Read the model definition and answer for the solid it produces. Units are mm, in the model's axes. Face numbers are marked on the shaded views. A direction names the side the tool comes from. Coordinates: 2 decimals unless noted, no trailing zeros. Write each loop counter-clockwise with the first axis right and the second up, starting at its lowest first coordinate (ties: lowest second). Pieces come first, ordered by that corner, then holes. Notation, with made-up numbers: M 41,-21 L 82,-21 A22 cw 82,9 Z; hole C -19,-14 d5. An arc over 180 degrees is marked long. Use a Markdown table: item, result. Add a question column.
from build123d import *

# Parameters (mm, degrees)
SKETCH1_W                 = 71
SKETCH1_H                 = 250
BOSS_EXTRUDE1_DEPTH       = 5
SKETCH2_W                 = 65
SKETCH2_H                 = 45
BOSS_EXTRUDE3_DEPTH       = 2
LPATTERN1_COUNT           = 3
LPATTERN1_PITCH           = 50
SKETCH3_W                 = 69
SKETCH3_H                 = 48.754858224
BOSS_EXTRUDE8_DEPTH       = 25
LPATTERN5_COUNT           = 3
LPATTERN5_PITCH           = 50
LPATTERN6_COUNT           = 3
LPATTERN6_PITCH           = 70
LPATTERN6_COPY_1_SKETCH_W = 65
LPATTERN6_COPY_1_SKETCH_H = 45
LPATTERN6_COPY_1_DEPTH    = 2
LPATTERN6_COPY_2_SKETCH_W = 65
LPATTERN6_COPY_2_SKETCH_H = 45
LPATTERN6_COPY_2_DEPTH    = 2
LPATTERN6_COPY_3_SKETCH_W = 65
LPATTERN6_COPY_3_SKETCH_H = 45
LPATTERN6_COPY_3_DEPTH    = 2
LPATTERN6_COPY_4_SKETCH_W = 65
LPATTERN6_COPY_4_SKETCH_H = 45
LPATTERN6_COPY_4_DEPTH    = 2
LPATTERN6_COPY_5_SKETCH_W = 69
LPATTERN6_COPY_5_SKETCH_H = 48.754858224
LPATTERN6_COPY_5_DEPTH    = 25
LPATTERN6_COPY_6_SKETCH_W = 69
LPATTERN6_COPY_6_SKETCH_H = 48.754858224
LPATTERN6_COPY_6_DEPTH    = 25
LPATTERN6_COPY_7_SKETCH_W = 69
LPATTERN6_COPY_7_SKETCH_H = 48.754858224
LPATTERN6_COPY_7_DEPTH    = 25
LPATTERN6_COPY_8_SKETCH_W = 69
LPATTERN6_COPY_8_SKETCH_H = 48.754858224
LPATTERN6_COPY_8_DEPTH    = 25
SKETCH6_W                 = 211
SKETCH6_H                 = 98.778316014
CUT_EXTRUDE1_DEPTH        = 10


with BuildPart() as part:
    # Sketch1 → Boss-Extrude1 (new body)
    with BuildSketch(Plane(origin=(0, 0, 0), x_dir=(1, 0, 0), z_dir=(0, 1, 0))):
        Rectangle(SKETCH1_W, SKETCH1_H)
    boss_extrude1 = extrude(amount=BOSS_EXTRUDE1_DEPTH)

    # Sketch2 → Boss-Extrude3 (add)
    with BuildSketch(Plane(origin=(0, 5, 0), x_dir=(1, 0, 0), z_dir=(0, 1, 0))):
        with Locations((0, -100)):
            Rectangle(SKETCH2_W, SKETCH2_H)
    boss_extrude3 = extrude(amount=BOSS_EXTRUDE3_DEPTH)

    # LPattern1: Boss-Extrude3 ×3
    with Locations(*[(0, 0, -i * LPATTERN1_PITCH) for i in range(1, LPATTERN1_COUNT)]):
        add(boss_extrude3)

    # Sketch3 → Boss-Extrude8 (add)
    with BuildSketch(Plane(origin=(0, 7, 0), x_dir=(1, 0, 0), z_dir=(0, 1, 0))):
        with Locations((0, -99.635002086)):
            Rectangle(SKETCH3_W, SKETCH3_H)
    boss_extrude8 = extrude(amount=BOSS_EXTRUDE8_DEPTH)

    # LPattern5: Boss-Extrude8 ×3
    with Locations(*[(0, 0, -i * LPATTERN5_PITCH) for i in range(1, LPATTERN5_COUNT)]):
        add(boss_extrude8)

    # LPattern6: Boss-Extrude1, Boss-Extrude3, Boss-Extrude8 ×3
    with Locations(*[(i * LPATTERN6_PITCH, 0, 0) for i in range(1, LPATTERN6_COUNT)]):
        add(boss_extrude1)
        add(boss_extrude3)
        add(boss_extrude8)

    # LPattern6 copy 1 sketch → LPattern6 copy 1 (add)
    with BuildSketch(Plane(origin=(70, 5, -50), x_dir=(1, 0, 0), z_dir=(0, 1, 0))):
        with Locations((0, -100)):
            Rectangle(LPATTERN6_COPY_1_SKETCH_W, LPATTERN6_COPY_1_SKETCH_H)
    extrude(amount=LPATTERN6_COPY_1_DEPTH)

    # LPattern6 copy 2 sketch → LPattern6 copy 2 (add)
    with BuildSketch(Plane(origin=(140, 5, -50), x_dir=(1, 0, 0), z_dir=(0, 1, 0))):
        with Locations((0, -100)):
            Rectangle(LPATTERN6_COPY_2_SKETCH_W, LPATTERN6_COPY_2_SKETCH_H)
    extrude(amount=LPATTERN6_COPY_2_DEPTH)

    # LPattern6 copy 3 sketch → LPattern6 copy 3 (add)
    with BuildSketch(Plane(origin=(70, 5, -100), x_dir=(1, 0, 0), z_dir=(0, 1, 0))):
        with Locations((0, -100)):
            Rectangle(LPATTERN6_COPY_3_SKETCH_W, LPATTERN6_COPY_3_SKETCH_H)
    extrude(amount=LPATTERN6_COPY_3_DEPTH)

    # LPattern6 copy 4 sketch → LPattern6 copy 4 (add)
    with BuildSketch(Plane(origin=(140, 5, -100), x_dir=(1, 0, 0), z_dir=(0, 1, 0))):
        with Locations((0, -100)):
            Rectangle(LPATTERN6_COPY_4_SKETCH_W, LPATTERN6_COPY_4_SKETCH_H)
    extrude(amount=LPATTERN6_COPY_4_DEPTH)

    # LPattern6 copy 5 sketch → LPattern6 copy 5 (add)
    with BuildSketch(Plane(origin=(70, 7, -50), x_dir=(1, 0, 0), z_dir=(0, 1, 0))):
        with Locations((0, -99.635002086)):
            Rectangle(LPATTERN6_COPY_5_SKETCH_W, LPATTERN6_COPY_5_SKETCH_H)
    extrude(amount=LPATTERN6_COPY_5_DEPTH)

    # LPattern6 copy 6 sketch → LPattern6 copy 6 (add)
    with BuildSketch(Plane(origin=(140, 7, -50), x_dir=(1, 0, 0), z_dir=(0, 1, 0))):
        with Locations((0, -99.635002086)):
            Rectangle(LPATTERN6_COPY_6_SKETCH_W, LPATTERN6_COPY_6_SKETCH_H)
    extrude(amount=LPATTERN6_COPY_6_DEPTH)

    # LPattern6 copy 7 sketch → LPattern6 copy 7 (add)
    with BuildSketch(Plane(origin=(70, 7, -100), x_dir=(1, 0, 0), z_dir=(0, 1, 0))):
        with Locations((0, -99.635002086)):
            Rectangle(LPATTERN6_COPY_7_SKETCH_W, LPATTERN6_COPY_7_SKETCH_H)
    extrude(amount=LPATTERN6_COPY_7_DEPTH)

    # LPattern6 copy 8 sketch → LPattern6 copy 8 (add)
    with BuildSketch(Plane(origin=(140, 7, -100), x_dir=(1, 0, 0), z_dir=(0, 1, 0))):
        with Locations((0, -99.635002086)):
            Rectangle(LPATTERN6_COPY_8_SKETCH_W, LPATTERN6_COPY_8_SKETCH_H)
    extrude(amount=LPATTERN6_COPY_8_DEPTH)

    # Sketch6 → Cut-Extrude1 (cut)
    with BuildSketch(Plane(origin=(0, 5, 0), x_dir=(1, 0, 0), z_dir=(0, 1, 0))):
        with Locations((70, 75.610841993)):
            Rectangle(SKETCH6_W, SKETCH6_H)
    extrude(amount=-CUT_EXTRUDE1_DEPTH, mode=Mode.SUBTRACT)


solid = part.part
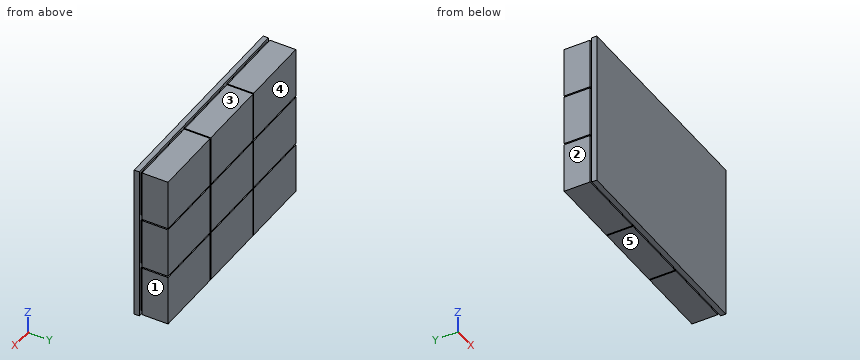
Item 1: Each of these flat-tipped pins is pushed along its axis until it touches: pin 1 (3 mm diameter, centred on y = 17, z = 95, fed in from -X); pin 2 (2 mm diameter, centred on x = 97, y = 24.5, fed in from +Z); pin 3 (1 mm diameter, centred on x = -6.5, y = 6, fed in from +Z). Where does it stop, or does it pass through?
Item 2: Find section C-C on y = 27.5. Count the separate pieces of the cut face and the enclosed holes in it, then the cut area to 3 significant figures.
Item 3: Find section A-A on x = -20. Give the vertices of the cut face in (y, z).
Item 4: Find section B-B on z = 9.5. Give the vertices of the cut face in (x, y), then the cut area to 3 significant figures.
Item 5: Consider probe 1 along Z at (x, y) = (17, 30); probe 2 along X at (y, z) = (16, 119); probe 3 along Z at (x, y) = (16, 5.5). Determine where each line is inside the solid, lowest interval first.
Item 6: For the marked faces 1, 2, 3, 4 and 5, determine the directions among +Z, -Z, +X, -X, +Y, -Y from which every point of the face is accessible in a straight line to the end or side of a thin tool.
Geometry says:
| question | item | result |
|---|---|---|
| 1 | pin 1 | stops at x = -34.5 |
| 1 | pin 2 | stops at z = 124.01 |
| 1 | pin 3 | stops at z = 122.5 |
| 2 | separate pieces | 9 |
| 2 | enclosed holes | 0 |
| 2 | area | 30,300 mm2 |
| 3 | outline | M 0,-26.22 L 5,-26.22 L 5,-22.5 L 7,-22.5 L 7,-24.74 L 32,-24.74 L 32,24.01 L 7,24.01 L 7,22.5 L 5,22.5 L 5,27.5 L 7,27.5 L 7,25.26 L 32,25.26 L 32,74.01 L 7,74.01 L 7,72.5 L 5,72.5 L 5,77.5 L 7,77.5 L 7,75.26 L 32,75.26 L 32,124.01 L 7,124.01 L 7,122.5 L 5,122.5 L 5,125 L 0,125 Z |
| 4 | outline | M -35.5,0 L 175.5,0 L 175.5,5 L 172.5,5 L 172.5,7 L 174.5,7 L 174.5,32 L 105.5,32 L 105.5,7 L 107.5,7 L 107.5,5 L 102.5,5 L 102.5,7 L 104.5,7 L 104.5,32 L 35.5,32 L 35.5,7 L 37.5,7 L 37.5,5 L 32.5,5 L 32.5,7 L 34.5,7 L 34.5,32 L -34.5,32 L -34.5,7 L -32.5,7 L -32.5,5 L -35.5,5 Z |
| 4 | area | 6,620 mm2 |
| 5 | probe 1 | z = -24.74 to 24.01, 25.26 to 74.01, 75.26 to 124.01 |
| 5 | probe 2 | x = -34.5 to 34.5, 35.5 to 104.5, 105.5 to 174.5 |
| 5 | probe 3 | z = -22.5 to 22.5, 27.5 to 72.5, 77.5 to 122.5 |
| 6 | face 1 | +Z, -Z, +X, +Y |
| 6 | face 2 | +Z, -Z, -X, +Y |
| 6 | face 3 | +Z, +X, -X, +Y |
| 6 | face 4 | +Z, -Z, +X, -X, +Y |
| 6 | face 5 | -Z, +X, -X, +Y |
